from build123d import *

# Parameters (mm, degrees)
SKETCH_1_W      = 32
SKETCH_1_H      = 16
SKETCH_1_R      = 1.25
EXTRUDE_1_DEPTH = 1.5
EXTRUDE_2_DEPTH = 1
FILLET_2_R      = 0.3


with BuildPart() as part:
    # Эскиз1 → Бобышка-Вытянуть1 (new body)
    with BuildSketch(Plane.XY):
        Rectangle(SKETCH_1_W, SKETCH_1_H)
        with Locations((-13, 0)):
            Circle(SKETCH_1_R, mode=Mode.SUBTRACT)
        with Locations((13, 0)):
            Circle(SKETCH_1_R, mode=Mode.SUBTRACT)
    extrude(amount=EXTRUDE_1_DEPTH)

    # Эскиз3 → Бобышка-Вытянуть2 (add)
    # profile 1 of 4: a face of its own
    with BuildSketch(Plane.XY.offset(1.5)):
        Polygon((-11, 4), (-11, -4), (-9.5, -4), (-9.5, -0.217121743), (-8, -0.217121743), (-8, -4), (-6.5, -4), (-6.5, 4), (-8, 4), (-8, 0.55188973), (-9.5, 0.55188973), (-9.5, 4), align=None)
    # profile 2 of 4: a face of its own
    with BuildSketch(Plane.XY.offset(1.5)):
        Polygon((-5.3, 4), (-5.3, -4), (0.67028136, -3.446242786), (0.67028136, 3.084011942), align=None)
        Polygon((-3.8, 2.252311448), (-3.8, -2.317138921), (-0.82971864, -2.041638549), (-0.82971864, 1.796597204), align=None, mode=Mode.SUBTRACT)
    # profile 3 of 4: a face of its own
    with BuildSketch(Plane.XY.offset(1.5)):
        Polygon((1.87028136, 4), (1.87028136, -4), (3.37028136, -4), (3.37028136, 1.197224362), (4.87028136, 0.197224362), (6.37028136, 1.197224362), (6.37028136, -4), (7.87028136, -4), (7.87028136, 4), (4.87028136, 2), align=None)
    # profile 4 of 4: a face of its own
    with BuildSketch(Plane.XY.offset(1.5)):
        Polygon((9.07028136, 4), (12.17028136, 4), (12.17028136, 2.5), (11.37028136, 2.5), (11.37028136, -2.5), (12.17028136, -2.5), (12.17028136, -4), (9.07028136, -4), (9.07028136, -2.5), (9.87028136, -2.5), (9.87028136, 2.5), (9.07028136, 2.5), align=None)
    extrude(amount=EXTRUDE_2_DEPTH)

    # Скругление2
    fillet_2_edges = [part.edges().sort_by_distance(p)[0] for p in [
        (16, 0, 1.5),
        (9.07028136, 3.25, 2.5),
        (9.47028136, 2.5, 2.5),
        (9.87028136, 0, 2.5),
        (9.47028136, -2.5, 2.5),
        (9.07028136, -3.25, 2.5),
        (10.62028136, -4, 2.5),
        (12.17028136, -3.25, 2.5),
        (11.77028136, -2.5, 2.5),
        (11.37028136, 0, 2.5),
        (11.77028136, 2.5, 2.5),
        (12.17028136, 3.25, 2.5),
        (10.62028136, 4, 2.5),
        (0, 8, 1.5),
        (-10.25, 4, 2.5),
        (-11, 0, 2.5),
        (-10.25, -4, 2.5),
        (-9.5, -2.108560871, 2.5),
        (-8.75, -0.217121743, 2.5),
        (-8, -2.108560871, 2.5),
        (-7.25, -4, 2.5),
        (-6.5, 0, 2.5),
        (-7.25, 4, 2.5),
        (-8, 2.275944865, 2.5),
        (-8.75, 0.55188973, 2.5),
        (-9.5, 2.275944865, 2.5),
        (-16, 0, 1.5),
        (-2.31485932, 3.542005971, 2.5),
        (-5.3, 0, 2.5),
        (-2.31485932, -3.723121393, 2.5),
        (0.67028136, -0.181115422, 2.5),
        (-2.31485932, 2.024454326, 2.5),
        (-3.8, -0.032413737, 2.5),
        (-2.31485932, -2.179388735, 2.5),
        (-0.82971864, -0.122520673, 2.5),
        (0, -8, 1.5),
        (2.62028136, -4, 2.5),
        (3.37028136, -1.401387819, 2.5),
        (4.12028136, 0.697224362, 2.5),
        (5.62028136, 0.697224362, 2.5),
        (6.37028136, -1.401387819, 2.5),
        (7.12028136, -4, 2.5),
        (7.87028136, 0, 2.5),
        (6.37028136, 3, 2.5),
        (3.37028136, 3, 2.5),
        (1.87028136, 0, 2.5),
    ]]
    fillet(fillet_2_edges, radius=FILLET_2_R)


solid = part.part
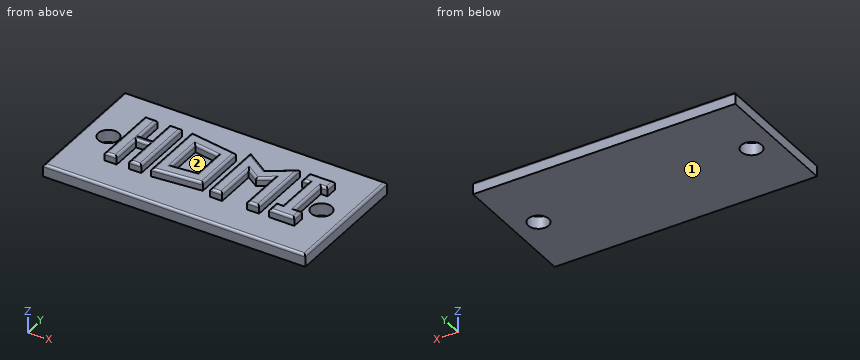
Read the model definition and answer for the solid it produces. Units are mm, in the model's axes. Face numbers are marked on the shaded views. Coordinates: 2 decimals unless noted, no trailing zeros. Loops run counter-clockwise (first coordinate to the right, second up) from the corner with the lowest first, then second, coordinate; pieces in that order, holes last. Notation, with made-up numbers: (9, 19) -> (18, 19) arc R16 cw to (18, 28) -> close; hole circle Ø5 at (41, -31.75). An arc over 180 degrees is marked (long way). Answer in a Markdown table with one row per item.
Item 1: A cutting plane is placed at B-B on z = 0.8. Determine the outline of the cut face in (x, y), plus the area to 3 significant figures.
Returned:
| item | result |
|---|---|
| outline | (-16, -8) -> (16, -8) -> (16, 8) -> (-16, 8) -> close; hole circle Ø2.5 at (-13, 0); hole circle Ø2.5 at (13, 0) |
| area | 502 mm^2 |
Item 2: Each of these flat-tipped pins is pushed along its axis until it touches: P1, Ø0.6, axis at y = -0.5, z = 2, coming from the +X side; P2, Ø0.6, axis at x = -10.5, z = 2, coming from the +Y side; P3, Ø0.8, axis at y = 2.5, z = 2, coming from the -X side. Where does it stop, or does it pass through?
Returned:
| item | result |
|---|---|
| P1 | stops at x = 11.37 |
| P2 | stops at y = 4 |
| P3 | stops at x = -11 |
Item 3: A cutting plane is placed at A-A on x = -13. Determine the outline of the cut face in (y, z), plus the area to 3 significant figures.
Returned:
| item | result |
|---|---|
| outline | (-8, 0) -> (-1.25, 0) -> (-1.25, 1.5) -> (-7.7, 1.5) arc R0.3 ccw to (-8, 1.2) -> close; (1.25, 0) -> (8, 0) -> (8, 1.2) arc R0.3 ccw to (7.7, 1.5) -> (1.25, 1.5) -> close |
| area | 20.2 mm^2 |
Item 4: For a pull along X with two mould halves and no side action, classify the marked faces 1 and 2 as released by +X, released by -X, zero draft, split by the parting line, or undercut.
Returned:
| item | result |
|---|---|
| face 1 | zero draft |
| face 2 | undercut |
Item 5: Straight lines are drawn through the part: line 1 along Y through (x, z) = (-13, 0.7); line 2 along Z through (x, y) = (-13, -6); line 3 along Y through (x, z) = (12, 0.4). For each, find the intervals that lie inside material, in ascending order. Write a range as [from, to].
Returned:
| item | result |
|---|---|
| line 1 | y = [-8, -1.25], [1.25, 8] |
| line 2 | z = [0, 1.5] |
| line 3 | y = [-8, -0.75], [0.75, 8] |
Item 6: A cutting plane is placed at C-C on y = -6.5. Determine the outline of the cut face in (x, z), plus the area to 3 significant figures.
Returned:
| item | result |
|---|---|
| outline | (-16, 0) -> (16, 0) -> (16, 1.2) arc R0.3 ccw to (15.7, 1.5) -> (-15.7, 1.5) arc R0.3 ccw to (-16, 1.2) -> close |
| area | 48.0 mm^2 |
